```python
from build123d import *

# Parameters (mm, degrees)
F0_R      = 4.4
F1_DEPTH  = 20
F2_R      = 0.5
F4_R      = 7
F5_DEPTH  = 12
F6_W      = 0.4
F6_H      = 2
F7_DEPTH  = 5.8
F8_SIZE2  = 0.99999
F8_SIZE   = 2.59999
F9_R      = 7
F9_R_2    = 6.25
F10_DEPTH = 10


# Not quite as in the source:
# - a fillet or chamfer is up to 0.001 mm smaller than in the source, because OpenCascade refuses the exact size


with BuildPart() as f1:
    # F0 (on Top) → F1 (new body)
    with BuildSketch(Plane.XY):
        Circle(F0_R)
    extrude(amount=F1_DEPTH)

    # F2
    f2_edges = [f1.edges().sort_by_distance(p)[0] for p in [
        (-4.4, 0, 20),
        (-4.4, 0, 0),
    ]]
    fillet(f2_edges, radius=F2_R)

    # F4 (on offset) → F5 (join)
    with BuildSketch(Plane.XY.offset(17)):
        Circle(F4_R)
    extrude(amount=-F5_DEPTH)

    # F6 (on face) → F7 (join)
    with BuildSketch(Plane(origin=(0, 0, 0), x_dir=(1, 0, 0), z_dir=(0, 0, -1))):
        with Locations((-2.2, 0)):
            Rectangle(F6_W, F6_H)
        with Locations((2.2, 0)):
            Rectangle(F6_W, F6_H)
    extrude(amount=F7_DEPTH)

    # F8 (size 2.6 and 1 in the source; OpenCascade refuses exactly that, so slightly less here)
    f8_edges = [f1.edges().sort_by_distance(p)[0] for p in [
        (-7, 0, 17),
    ]]
    f8_side = f1.faces().sort_by_distance((-6.80201, 0, 17))[0]
    chamfer(f8_edges, length=F8_SIZE, length2=F8_SIZE2, reference=f8_side)

    # F9 (on face) → F10 (cut)
    with BuildSketch(Plane(origin=(0, 0, 5), x_dir=(1, 0, 0), z_dir=(0, 0, -1))):
        Circle(F9_R)
        Circle(F9_R_2, mode=Mode.SUBTRACT)
    extrude(amount=-F10_DEPTH, mode=Mode.SUBTRACT)


solid = f1.part
```
Read the model definition and answer for the solid it produces. Units are mm, in the model's axes. A direction names the side the tool comes from. Coordinates: 2 decimals unless noted, no trailing zeros. Loops run counter-clockwise (first coordinate to the right, second up) from the corner with the lowest first, then second, coordinate; pieces in that order, holes last. Notation, with made-up numbers: (-8.75, 60) - (38.25, 60) arc R24 ccw to (38.25, 70) - close; hole circle Ø4 at (78.5, 51.5). An arc over 180 degrees is marked (long way). Answer in a Markdown table with one row per item.
1. Determine the mould class of faces 4 (the face through (0, 0, 0)), 5 (the face through (2, 0, -3)), 6 (the face through (2.4, 0, -3)), 7 (the face through (6.466, -2.681, 15.507)) for opening direction X: +X half, -X half, draft (parallel to the pull), parting line (faces both ways), or undercut.
Conclusion:
| item | result |
|---|---|
| face 4 | undercut |
| face 5 | undercut |
| face 6 | +X half |
| face 7 | parting line |
2. Find section C-C, the plane z = 4.5. Write down the section's boundary in (x, y).
Conclusion:
| item | result |
|---|---|
| outline | circle Ø8.8 at (0, 0) |
3. Which of the six approach directions +Z, -Z, +X, -X, +Y, -Y give full straight-line access (tool end or side, diameter ignored) to faces 1 (the face through (-4.3, 1.5, 5)), 2 (the face through (4.197, 1.322, 18.232)), 3 (the face through (-2, 0, -3))?
Conclusion:
| item | result |
|---|---|
| face 1 | -Z |
| face 2 | +Z |
| face 3 | -Z, +Y, -Y |
4. Given pin 1 (4 mm diameter, centred on x = -4, y = -5.5, fed in from -Z); pin 2 (1 mm diameter, centred on x = -4, z = 3, fed in from -Y); pin 3 (3 mm diameter, centred on y = 0.5, z = 8, fed in from +X), each flat-ended and moving along its own axis, determine where each tip first touches the part or whether it passes through.
Conclusion:
| item | result |
|---|---|
| pin 1 | stops at z = 5 |
| pin 2 | stops at y = -2.67 |
| pin 3 | stops at x = 6.25 |
5. Straight lines are drawn through the part: line 1 (X direction, y = 0.5, z = -2.5); line 2 (Z direction, x = -3, y = -1); line 3 (X direction, y = 0.25, z = 14) (3 decimals). For each, find the intervals that lie inside material, in ascending order.
Conclusion:
| item | result |
|---|---|
| line 1 | x = -2.4 to -2, 2 to 2.4 |
| line 2 | z = 0 to 20 |
| line 3 | x = -6.245 to 6.245 |
